Check sheet for the drawn part. Datum: minimum x, y, z corner. Units: mm. A direction names the side the tool comes from. Give positions to 0.01 mm unless a question says otherwise; leave off trailing zeros. Order: outer loops, then holes, each group sorted by start corner. A loop starts at its lowest first (then second) coordinate and runs counter-clockwise, first axis right, second up. Notation, with made-up numbers: (69, 64.5) -> (81, 64.5) arc R28 ccw to (81, 83.5) -> close; hole circle Ø11 at (-5.75, 74). An arc over 180 degrees is marked (long way). Answer in a Markdown table with one row per item. Add a question column.
(1) Cross-section at C-C (z = 4.5). Record the cut outline in (x, y), then the cut area to 3 significant figures.
(2) Go/stop test with flat-tipped pins: pin 1 (1.5 mm diameter, centred on y = 46.5, z = 7.5, fed in from +X); pin 2 (3 mm diameter, centred on x = 57.5, z = 13.5, fed in from -Y); pin 3 (4 mm diameter, centred on x = 54.5, z = 14, fed in from +Y). Record where each tip stops, or that it passes through.
(3) Cross-section at B-B (x = 49.5). Record the cut outline in (y, z) (3 decimals).
(4) Cross-section at A-A (y = 42.5). Record the cut outline in (x, z) (3 decimals), then the cut area to 3 significant figures.
(5) Thickness scan on L1, parallel to Z at x = 6.5, y = 13 (3 decimals); L2, parallel to X at y = 27, z = 12.5; L3, parallel to Y at x = 71, z = 4.25. Record the ranges inside material, lowest first. Write a range as [from, to].
(6) Set-up check for the marked faces 1, 2 and 3: record each of +Z, -Z, +X, -X, +Y, -Y from which the full face is reachable in a straight line by a thin tool's end or side.
(7) Cross-section at D-D (y = 7). Record the cut outline in (x, z) (3 decimals), then the cut area to 3 significant figures.
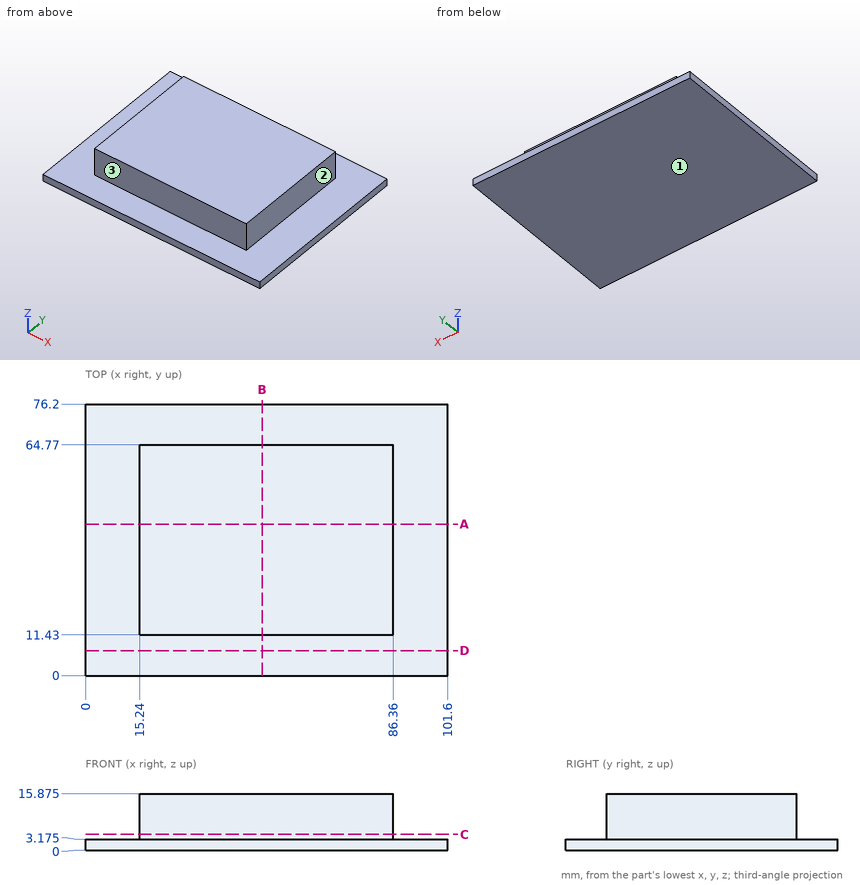
Answer below:
| question | item | result |
|---|---|---|
| 1 | outline | (15.24, 11.43) -> (86.36, 11.43) -> (86.36, 64.77) -> (15.24, 64.77) -> close |
| 1 | area | 3,790 mm² |
| 2 | pin 1 | stops at x = 86.36 |
| 2 | pin 2 | stops at y = 11.43 |
| 2 | pin 3 | stops at y = 64.77 |
| 3 | outline | (0, 0) -> (76.2, 0) -> (76.2, 3.175) -> (64.77, 3.175) -> (64.77, 15.875) -> (11.43, 15.875) -> (11.43, 3.175) -> (0, 3.175) -> close |
| 4 | outline | (0, 0) -> (101.6, 0) -> (101.6, 3.175) -> (86.36, 3.175) -> (86.36, 15.875) -> (15.24, 15.875) -> (15.24, 3.175) -> (0, 3.175) -> close |
| 4 | area | 1,230 mm² |
| 5 | L1 | z = [0, 3.175] |
| 5 | L2 | x = [15.24, 86.36] |
| 5 | L3 | y = [11.43, 64.77] |
| 6 | face 1 | -Z, +X, -X, +Y, -Y |
| 6 | face 2 | +Z, +X, +Y, -Y |
| 6 | face 3 | +Z, +X, -X, -Y |
| 7 | outline | (0, 0) -> (101.6, 0) -> (101.6, 3.175) -> (0, 3.175) -> close |
| 7 | area | 323 mm² |
